Read the model definition and answer for the solid it produces. Units are mm, in the model's axes. Face numbers are marked on the shaded views. A direction names the side the tool comes from. Give positions to 0.01 mm unless a question says otherwise; leave off trailing zeros. Write each loop counter-clockwise with the first axis right and the second up, starting at its lowest first coordinate (ties: lowest second). Pieces come first, ordered by that corner, then holes. Notation, with made-up numbers: (-8, 78) -> (37, 78) arc R18 cw to (37, 106) -> close; hole circle Ø8 at (-20.75, -23). An arc over 180 degrees is marked (long way). Use a Markdown table: item, result.
Autodesk Inventor part; units mm, degrees
ref_plane "YZ Plane" through (0, 0, 0) normal (1, 0, 0) x (0, 1, 0)
ref_plane "XZ Plane" through (0, 0, 0) normal (0, 1, 0) x (-1, 0, 0)
ref_plane "XY Plane" through (0, 0, 0) normal (0, 0, 1) x (1, 0, 0)
sketch "Sketch1" plane through (0, 0, 0) normal (0, 0, 1) x (1, 0, 0)
  line L0 (-21, 21) -> (21, 21)
  line L1 (21, 21) -> (21, -21)
  line L2 (21, -21) -> (-21, -21)
  line L3 (-21, -21) -> (-21, 21)
  line L4 (-21, 21) -> (21, -21) construction
  line L5 (21, 21) -> (-21, -21) construction
  circle A0 centre (15.5, 15.5) radius 1.6
  circle A1 centre (15.5, -15.5) radius 1.6
  line L6 (0, 0) -> (0, 3.2399) construction
  circle A2 centre (-15.5, 15.5) radius 1.6
  circle A3 centre (-15.5, -15.5) radius 1.6
  circle A4 centre (0, 0) radius 11.75
  line L7 (-25, 21) -> (25, 21)
  line L8 (25, 21) -> (25, -26)
  line L9 (25, -26) -> (-25, -26)
  line L10 (-25, -26) -> (-25, 21)
  dimension "d0" = 42
  dimension "d1" = 42
  dimension "d2" = 31
  dimension "d3" = 3.2
  dimension "d4" = 3.2
  dimension "d5" = 23.5
  dimension "d9" = 4
  dimension "d10" = 4
  dimension "d11" = 5
extrude "Extrusion1" add sketch "Sketch1" along normal blind 5.5
sketch "Sketch2" plane through (-25, -26, 0) normal (0, -1, 0) x (1, 0, 0)
  line L0 (0, 5.5) -> (50, 5.5)
  line L1 (50, 5.5) -> (0, 5.5)
  line L2 (0, 5.5) -> (0, -44.5)
  line L3 (0, -44.5) -> (50, -44.5)
  line L4 (50, -44.5) -> (50, 5.5)
  line L5 (0, 0) -> (0, 5.5)
  line L6 (0, 0) -> (50, -44.5) construction
  line L7 (50, 0) -> (0, -44.5) construction
  line L8 (50, 0) -> (0, 0)
  line L9 (8.4, -33.5) -> (41.6, -33.5) construction
  line L10 (10, -31.9) -> (40, -31.9)
  line L11 (40, -35.1) -> (10, -35.1)
  arc A0 (10, -31.9) -> (10, -35.1) centre (10, -33.5) ccw
  arc A1 (40, -35.1) -> (40, -31.9) centre (40, -33.5) ccw
  line L12 (8.4, -8.6) -> (41.6, -8.6) construction
  line L13 (10, -7) -> (40, -7)
  line L14 (40, -10.2) -> (10, -10.2)
  arc A2 (10, -7) -> (10, -10.2) centre (10, -8.6) ccw
  arc A3 (40, -10.2) -> (40, -7) centre (40, -8.6) ccw
  point P0 (25, 0)
  point P1 (49.9436, 3)
  point P2 (25, -33.5)
  point P3 (25, -8.6)
  dimension "d12" = 50
  dimension "d71" = 1.6
  dimension "d72" = 1.6
  dimension "d73" = 25
  dimension "d74" = 25
  dimension "d75" = 30
  dimension "d76" = 30
  dimension "d78" = 7
  dimension "d86" = 11
extrude "Extrusion2" add sketch "Sketch2" along normal blind 3
sketch "Sketch5" plane through (25, 21, 5.5) normal (1, 0, 0) x (0, 0, -1)
  line L0 (50, -47) -> (5.5, -47)
  line L1 (27.75, -47) -> (5.5, -24.75)
  line L2 (5.5, -47) -> (5.5, 0)
  point P0 (5.5, -21)
  dimension "d20" = 45
extrude "Extrusion3" add sketch "Sketch5" against normal blind 3.5
mirror "Mirror1" about plane through (0, 0, 0) normal (1, 0, 0) of "Extrusion3"
fillet "Fillet1" radius 2 7 edges at (0, -26, 0) (-21.5, -26, -11.125) (21.5, -26, -11.125) (23.25, -26, -22.25) (23.25, -3.75, 0) (-23.25, -3.75, 0) (-23.25, -26, -22.25)
fillet "Fillet2" radius 0.4 4 edges at (-20.9142, -25.4142, -0.5858) (-21.5, -13.875, 0) (20.9142, -25.4142, -0.5858) (21.5, -13.875, 0)
sketch "Sketch6" plane through (-25, -26, 0) normal (0, 1, 0) x (1, 0, 0)
  line L0 (0, -5.5) -> (0, 44.5)
  line L1 (50, 44.5) -> (50, -5.5)
  line L2 (0, 44.5) -> (50, 44.5)
  line L3 (50, 44.5) -> (50, 39.5)
  line L4 (50, 39.5) -> (0, 39.5)
  line L5 (0, 39.5) -> (0, 44.5)
  point P0 (25, 0)
  point P1 (0, 39.5)
  dimension "d25" = 5
extrude "Extrusion4" add sketch "Sketch6" along normal blind 5
fillet "Fillet3" radius 1.5 4 edges at (0, -21, -39.5) (0, -21, -44.5) (0, -26, -39.5) (0, -29, -44.5)
sketch "Sketch7" plane through (0, 0, 5.5) normal (0, 0, 1) x (1, 0, 0)
  line L0 (25, 21) -> (-25, 21)
  line L1 (-25, 21) -> (-25, -29)
  line L2 (25, -29) -> (-25, -29)
  line L3 (25, 21) -> (25, -29)
  circle A0 centre (15.5, 15.5) radius 1.6
  circle A1 centre (15.5, -15.5) radius 1.6
  circle A2 centre (-15.5, 15.5) radius 1.6
  circle A3 centre (-15.5, -15.5) radius 1.6
  circle A4 centre (0, 0) radius 11.75
  line L4 (35, 0) -> (-35, 0)
  line L5 (0, 0) -> (0, -3.907) construction
  line L6 (-12.4, -24.9) -> (12.4, -24.9)
  line L7 (12.4, -24.9) -> (12.4, -21.1)
  line L8 (12.4, -21.1) -> (-12.4, -21.1)
  line L9 (-12.4, -21.1) -> (-12.4, -24.9)
  line L10 (-12.4, -24.9) -> (12.4, -21.1) construction
  line L11 (12.4, -24.9) -> (-12.4, -21.1) construction
  circle A5 centre (-20, 0) radius 2.5
  circle A6 centre (-18, 10) radius 2.5
  circle A7 centre (-18, -10) radius 2.5
  circle A8 centre (18, -10) radius 2.5
  circle A9 centre (20, 0) radius 2.5
  circle A10 centre (18, 10) radius 2.5
  point P0 (0, -23)
  dimension "d94" = 3.8
  dimension "d95" = 23
  dimension "d96" = 24.8
  dimension "d97" = 12.4
  dimension "d98" = 5
  dimension "d99" = 5
  dimension "d100" = 5
  dimension "d101" = 10
  dimension "d102" = 10
  dimension "d103" = 2
  dimension "d104" = 2
  dimension "d105" = 20
extrude "Extrusion5" cut sketch "Sketch7" against normal up to surface (5.5 mm away) contours A9 L4 | L4 A9 | A5 L4 | L4 A5 | L9 L8 L7 L6 | A6 | A7 | A8 | A10
sketch "Sketch8" plane through (0, 0, 5.5) normal (0, 0, 1) x (1, 0, 0)
  circle A0 centre (-15.5, 15.5) radius 1.6
  circle A1 centre (15.5, 15.5) radius 1.6
  circle A2 centre (15.5, -15.5) radius 1.6
  circle A3 centre (-15.5, -15.5) radius 1.6
  point P0 (0, 0)
hole "Hole2" at (-15.5, 15.5, 5.5) at (15.5, 15.5, 5.5) at (15.5, -15.5, 5.5) at (-15.5, -15.5, 5.5) direction (0, 0, -1) diameter 3.2 depth 10 countersink diameter 6 countersink angle 90
chamfer "Chamfer1" distance 7 angle 45 2 edges at (-25, 21, 2.75) (25, 21, 2.75)
fillet "Fillet4" radius 1 1 edges at (0, -29, 5.5)
chamfer "Chamfer2" distance 1.125 angle 45 8 edges at (0, -26, -7) (16.6, -26, -8.6) (0, -26, -10.2) (-16.6, -26, -8.6) (0, -26, -31.9) (16.6, -26, -33.5) (0, -26, -35.1) (-16.6, -26, -33.5)
equation "\"d1\" = d0"
equation "\"d4\" = d3"
equation "\"d10\" = d9"
equation "\"d97\" = 0.5 * d96"
equation "\"d99\" = d98"
equation "\"d100\" = d99"
equation "\"d102\" = d101"
equation "\"d104\" = d103"
properties part number "Stepper Mount V4" material "Thermoplastic Resin"
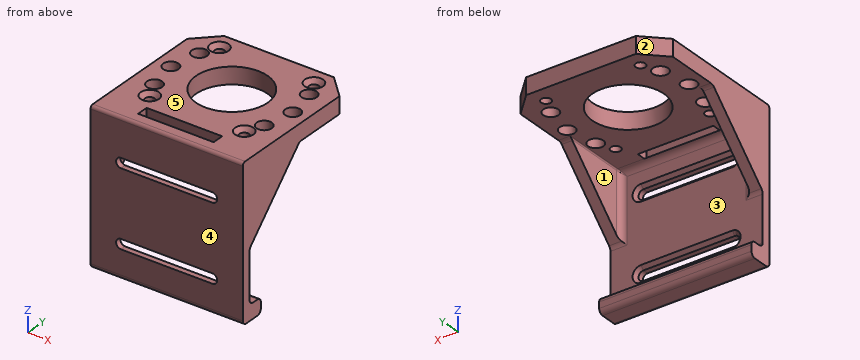
Item 1: A cutting plane is placed at D-D (y = -15.5). Give the vertices of the cut face in (x, z).
Return value:
| item | result |
|---|---|
| outline | (-25, -11.75) -> (-21.5, -11.75) -> (-21.5, -0.4) arc R0.4 cw to (-21.1, 0) -> (-17.1, 0) -> (-17.1, 4.1) -> (-18.5, 5.5) -> (-25, 5.5) -> close; (-13.9, 0) -> (13.9, 0) -> (13.9, 4.1) -> (12.5, 5.5) -> (-12.5, 5.5) -> (-13.9, 4.1) -> close; (17.1, 0) -> (21.1, 0) arc R0.4 cw to (21.5, -0.4) -> (21.5, -11.75) -> (25, -11.75) -> (25, 5.5) -> (18.5, 5.5) -> (17.1, 4.1) -> close |
Item 2: A tool of negligible diameter and unlimited length cuts with its end or side. For the marked faces 1 and 2, from which of +Z, -Z, +X, -X, +Y, -Y can it reach the whole face along a straight path? Write none if from no direction.
Return value:
| item | result |
|---|---|
| face 1 | +Y |
| face 2 | +Z, -Z, -X, +Y |
Item 3: Each of these flat-tipped pins is pushed along its axis until it touches: P1, Ø0.6, axis at x = -10, y = -23.5, coming from the +Z side; P2, Ø3.5, axis at x = 15.5, y = -15.5, coming from the +Z side; P3, Ø6, axis at x = 5.5, z = -10.5, coming from the +Y side. Where does it stop, or does it pass through?
Return value:
| item | result |
|---|---|
| P1 | z = -39.5 |
| P2 | z = 4.25 |
| P3 | y = -26 |
Item 4: A cutting plane is placed at B-B (x = 0). Count the separate pieces of the cut face and the enclosed holes in it, then the cut area to 3 significant figures.
Return value:
| item | result |
|---|---|
| separate pieces | 5 |
| enclosed holes | 0 |
| area | 261 mm^2 |
Item 5: A cutting plane is placed at C-C (z = -16.5). Give the vertices of the cut face in (x, y).
Return value:
| item | result |
|---|---|
| outline | (-25, -29) -> (25, -29) -> (25, -20.25) -> (21.5, -20.25) -> (21.5, -24) arc R2 cw to (19.5, -26) -> (-19.5, -26) arc R2 cw to (-21.5, -24) -> (-21.5, -20.25) -> (-25, -20.25) -> close |
Item 6: Straight lines are drawn through the part: line 1 along Y through (x, z) = (-20, 3); line 2 along Y through (x, z) = (15, 1); line 3 along Z through (x, y) = (-4, -19). For each, find the intervals that lie inside material, in ascending order. Write a range as [from, to].
Return value:
| item | result |
|---|---|
| line 1 | [-29, -11.5], [-8.5, -2.5], [2.5, 8.5], [11.5, 19] |
| line 2 | [-29, -17.02], [-13.98, 13.98], [17.02, 21] |
| line 3 | [0, 5.5] |
Item 7: For a pull along Z with two mould halves and no side action, classify the marked faces 3, 4 and 5 as +Z half, -Z half, draft (parallel to the pull), parting line (faces both ways), or undercut.
Return value:
| item | result |
|---|---|
| face 3 | undercut |
| face 4 | draft |
| face 5 | +Z half |
Item 8: A cutting plane is placed at A-A (y = 15.5). Give the vertices of the cut face in (x, z), then the cut area to 3 significant figures.
Return value:
| item | result |
|---|---|
| outline | (-23.5, 0) -> (-17.1, 0) -> (-17.1, 4.1) -> (-18.5, 5.5) -> (-23.5, 5.5) -> close; (-13.9, 0) -> (13.9, 0) -> (13.9, 4.1) -> (12.5, 5.5) -> (-12.5, 5.5) -> (-13.9, 4.1) -> close; (17.1, 0) -> (23.5, 0) -> (23.5, 5.5) -> (18.5, 5.5) -> (17.1, 4.1) -> close |
| area | 219 mm^2 |
